Geometry: final body of the model. Coordinates: model frame, mm. A direction names the side the tool comes from. Coordinates: 2 decimals unless noted, no trailing zeros. Loops run counter-clockwise (first coordinate to the right, second up) from the corner with the lowest first, then second, coordinate; pieces in that order, holes last. Notation, with made-up numbers: (-9, 59.5) - (15, 59.5) arc R24 cw to (15, 88.5) - close; hole circle Ø5 at (36, 14.25). An arc over 180 degrees is marked (long way). Return JSON: item names as keys, results as strings.
from build123d import *

# Parameters (mm, degrees)
F0_R     = 11.1125
F1_DEPTH = 53.34
F2_SIZE  = 5.08
F3_R     = 8.5725
F4_DEPTH = 50.8


with BuildPart() as f1:
    # F0 (on Front) → F1 (new body)
    with BuildSketch(Plane.XZ):
        with Locations((-37.678103, 0)):
            Circle(F0_R)
    extrude(amount=F1_DEPTH)

    # F2
    f2_edges = [f1.edges().sort_by_distance(p)[0] for p in [
        (-48.790603, -53.34, 0),
    ]]
    chamfer(f2_edges, length=F2_SIZE)

    # F3 (on face) → F4 (join)
    with BuildSketch(Plane.XZ):
        with Locations((-37.773054, 0)):
            Circle(F3_R)
    extrude(amount=-F4_DEPTH)


solid = f1.part
Item 1: Ray query, probe 1 along Z at (x, y) = (-37.75, 25); probe 2 along Z at (x, y) = (-37.5, -26); probe 3 along X at (y, z) = (9, -2.75). Return the intervals inside material, ascending. Write a range as from..to.
Worked out:
{"probe 1": "-8.57..8.57", "probe 2": "-11.11..11.11", "probe 3": "-45.89..-29.65"}
Item 2: Section query C-C, the plane y = 16.5. Return loops of the section in (x, z) (1 decimal), and give its area (3 significant figures).
Worked out:
{"outline": "circle Ø17.1 at (-37.8, 0)", "area": "231 mm^2"}
Item 3: Reachability of faces 1 (the face through (-48.78, -23.79, 0.49)), 2 (the face through (-33.165, 25.044, 7.228)) from +Z, -Z, +X, -X, +Y, -Y: full face, straight path, thin tool, end or side. Return the list, or none.
Worked out:
{"face 1": "+Y, -Y", "face 2": "+Y"}
Item 4: Section query B-B, the plane y = -40.5. Return loops of the section in (x, z) (1 decimal), and give its area (3 significant figures).
Worked out:
{"outline": "circle Ø22.2 at (-37.7, 0)", "area": "388 mm^2"}
Item 5: First-contact query: pin 1 Ø6 at (y, z) = (39, 4) entering from +X; pin 2 Ø8 at (y, z) = (-17, 8.5) entering from -X; pin 3 Ø1 at (y, z) = (25.5, -0.5) entering from -X; pin 4 Ø12 at (x, y) = (-43, -39) entering from -Z. Flat tips, straight axial feed; report the tip coordinate or a pass-through.
Worked out:
{"pin 1": "x = -29.26", "pin 2": "x = -47.84", "pin 3": "x = -46.35", "pin 4": "z = -11.11"}
Item 6: Section query A-A, the plane z = 0. Return loops of the section in (x, y), and give its area (3 significant figures).
Worked out:
{"outline": "(-48.79, -48.26) - (-43.71, -53.34) - (-31.65, -53.34) - (-26.57, -48.26) - (-26.57, 0) - (-29.2, 0) - (-29.2, 50.8) - (-46.35, 50.8) - (-46.35, 0) - (-48.79, 0) - close", "area": "2,030 mm^2"}
